from build123d import *

# Parameters (mm, degrees)
ESQUISSE1_W             = 51.75
ESQUISSE1_H             = 25.15
BOSS_EXTRU_1_DEPTH      = 1.25
ENL_V_MAT_EXTRU_1_DEPTH = 1.25
ESQUISSE3_R             = 0.762
ENL_V_MAT_EXTRU_2_DEPTH = 1.25
ESQUISSE4_W             = 34.186682017
ESQUISSE4_H             = 20.933463699
BOSS_EXTRU_2_DEPTH      = 2.3


with BuildPart() as part:
    # Esquisse1 → Boss.-Extru.1 (new body)
    with BuildSketch(Plane(origin=(0, 0, 0), x_dir=(1, 0, 0), z_dir=(0, 1, 0))):
        with Locations((25.875, 12.575)):
            Rectangle(ESQUISSE1_W, ESQUISSE1_H)
    extrude(amount=BOSS_EXTRU_1_DEPTH)

    # Esquisse2 → Enlèv. mat.-Extru.1 (cut)
    with BuildSketch(Plane(origin=(0, 1.25, 0), x_dir=(1, 0, 0), z_dir=(0, 1, 0))):
        Polygon((0, 25.15), (2.45, 25.15), (0, 22.7), align=None)
        Polygon((0, 0), (2.45, 0), (0, 2.45), align=None)
    extrude(amount=-ENL_V_MAT_EXTRU_1_DEPTH, mode=Mode.SUBTRACT)

    # Esquisse3 → Enlèv. mat.-Extru.2 (cut)
    with BuildSketch(Plane(origin=(0, 1.25, 0), x_dir=(1, 0, 0), z_dir=(0, 1, 0))):
        with Locations((3.38, 24.26)):
            Circle(ESQUISSE3_R)
        with Locations((5.92, 24.26)):
            Circle(ESQUISSE3_R)
        with Locations((8.46, 24.26)):
            Circle(ESQUISSE3_R)
        with Locations((11, 24.26)):
            Circle(ESQUISSE3_R)
        with Locations((13.54, 24.26)):
            Circle(ESQUISSE3_R)
        with Locations((16.08, 24.26)):
            Circle(ESQUISSE3_R)
        with Locations((18.62, 24.26)):
            Circle(ESQUISSE3_R)
        with Locations((21.16, 24.26)):
            Circle(ESQUISSE3_R)
        with Locations((23.7, 24.26)):
            Circle(ESQUISSE3_R)
        with Locations((26.24, 24.26)):
            Circle(ESQUISSE3_R)
        with Locations((28.78, 24.26)):
            Circle(ESQUISSE3_R)
        with Locations((31.32, 24.26)):
            Circle(ESQUISSE3_R)
        with Locations((33.86, 24.26)):
            Circle(ESQUISSE3_R)
        with Locations((36.4, 24.26)):
            Circle(ESQUISSE3_R)
        with Locations((38.94, 24.26)):
            Circle(ESQUISSE3_R)
        with Locations((41.48, 24.26)):
            Circle(ESQUISSE3_R)
        with Locations((44.02, 24.26)):
            Circle(ESQUISSE3_R)
        with Locations((46.56, 24.26)):
            Circle(ESQUISSE3_R)
        with Locations((46.56, 0.89)):
            Circle(ESQUISSE3_R)
        with Locations((44.02, 0.89)):
            Circle(ESQUISSE3_R)
        with Locations((41.48, 0.89)):
            Circle(ESQUISSE3_R)
        with Locations((38.94, 0.89)):
            Circle(ESQUISSE3_R)
        with Locations((36.4, 0.89)):
            Circle(ESQUISSE3_R)
        with Locations((33.86, 0.89)):
            Circle(ESQUISSE3_R)
        with Locations((31.32, 0.89)):
            Circle(ESQUISSE3_R)
        with Locations((28.78, 0.89)):
            Circle(ESQUISSE3_R)
        with Locations((26.24, 0.89)):
            Circle(ESQUISSE3_R)
        with Locations((23.7, 0.89)):
            Circle(ESQUISSE3_R)
        with Locations((18.62, 0.89)):
            Circle(ESQUISSE3_R)
        with Locations((21.16, 0.89)):
            Circle(ESQUISSE3_R)
        with Locations((16.08, 0.89)):
            Circle(ESQUISSE3_R)
        with Locations((13.54, 0.89)):
            Circle(ESQUISSE3_R)
        with Locations((11, 0.89)):
            Circle(ESQUISSE3_R)
        with Locations((8.46, 0.89)):
            Circle(ESQUISSE3_R)
        with Locations((5.92, 0.89)):
            Circle(ESQUISSE3_R)
        with Locations((3.38, 0.89)):
            Circle(ESQUISSE3_R)
    extrude(amount=-ENL_V_MAT_EXTRU_2_DEPTH, mode=Mode.SUBTRACT)

    # Esquisse4 → Boss.-Extru.2 (add)
    with BuildSketch(Plane(origin=(0, 1.25, 0), x_dir=(1, 0, 0), z_dir=(0, 1, 0))):
        with Locations((31.885763085, 12.597978811)):
            Rectangle(ESQUISSE4_W, ESQUISSE4_H)
    extrude(amount=BOSS_EXTRU_2_DEPTH)


solid = part.part
Design review of the part built by this model. Coordinates are the model's own, in mm. A direction names the side the tool comes from. Coordinates: 2 decimals unless noted, no trailing zeros. Loops run counter-clockwise (first coordinate to the right, second up) from the corner with the lowest first, then second, coordinate; pieces in that order, holes last. Notation, with made-up numbers: (-29.5, 88.5) -> (11.5, 88.5) arc R25 ccw to (11.5, 120.5) -> close; hole circle Ø11 at (-4, 30). An arc over 180 degrees is marked (long way). Use a Markdown table: item, result. Add a question column.
Item 1: We need section D-D, the plane z = -24.26. Count the separate pieces of the cut face and the enclosed holes in it, and give its area (3 significant figures).
Item 2: We need section B-B, the plane z = -12.75. Write out the cut boundary in (x, y), and give its area (3 significant figures).
Item 3: We need section C-C, the plane x = 5.92. Write out the cut boundary in (y, z), and give its area (3 significant figures).
Item 4: Machinability: for faces 4 (the flat face through (32, 2, -23.065)), 5 (the cylindrical face through (38.18, 0.63, -0.92)), 6 (the flat face through (14.792, 2, -12)), which of the approach directions +Z, -Z, +X, -X, +Y, -Y give a long, thin tool a straight path to every point of the face, cutting with its end or side? Answer none if there is none.
Item 5: We need section A-A, the plane x = 23.7. Write out the cut boundary in (y, z), and give its area (3 significant figures).
Item 6: Wall thickness on L1, parallel to X at y = 1.8, z = -14.75; L2, parallel to Y at x = 8, z = -23; L3, parallel to Z at x = 23.5, y = 3.15: over which ranges is each line inside the solid? List them lowest first. Write a range as from..to.
Item 7: Clearance check with flat-ended pins moving along their axes: P1, Ø2, axis at x = 16.08, z = -24.26, coming from the +Y side; P2, Ø1.8, axis at x = 30, y = 2.5, coming from the +Z side. State where each tip first meets the part, or that it passes through.
Item 8: The part is to be moulded in two halves that separate along X. For faces 1 (the flat face through (1.24, 0.63, -1.21)), 2 (the flat face through (51.75, 1, -12)), 3 (the cylindrical face through (5.16, 0.63, -0.92)), say which applies: +X half, -X half, draft (parallel to the pull), parting line (faces both ways), or undercut.
Numbers:
| question | item | result |
|---|---|---|
| 1 | separate pieces | 19 |
| 1 | enclosed holes | 0 |
| 1 | area | 28.4 mm^2 |
| 2 | outline | (0, 0) -> (51.75, 0) -> (51.75, 1.25) -> (48.98, 1.25) -> (48.98, 3.55) -> (14.79, 3.55) -> (14.79, 1.25) -> (0, 1.25) -> close |
| 2 | area | 143 mm^2 |
| 3 | outline | (0, -25.15) -> (1.25, -25.15) -> (1.25, -25.02) -> (0, -25.02) -> close; (0, -23.5) -> (1.25, -23.5) -> (1.25, -1.65) -> (0, -1.65) -> close; (0, -0.13) -> (1.25, -0.13) -> (1.25, 0) -> (0, 0) -> close |
| 3 | area | 27.6 mm^2 |
| 4 | face 4 | -Z, +X, -X, +Y |
| 4 | face 5 | +Y, -Y |
| 4 | face 6 | +Z, -Z, -X, +Y |
| 5 | outline | (0, -25.15) -> (1.25, -25.15) -> (1.25, -25.02) -> (0, -25.02) -> close; (0, -23.5) -> (1.25, -23.5) -> (1.25, -23.06) -> (3.55, -23.06) -> (3.55, -2.13) -> (1.25, -2.13) -> (1.25, -1.65) -> (0, -1.65) -> close; (0, -0.13) -> (1.25, -0.13) -> (1.25, 0) -> (0, 0) -> close |
| 5 | area | 75.8 mm^2 |
| 6 | L1 | x = 14.79..48.98 |
| 6 | L2 | y = 0..1.25 |
| 6 | L3 | z = -23.06..-2.13 |
| 7 | P1 | stops at y = 1.25 |
| 7 | P2 | stops at z = -2.13 |
| 8 | face 1 | -X half |
| 8 | face 2 | +X half |
| 8 | face 3 | undercut |
